Here's how the part is built. I have some questions about the finished solid (model axes, mm). A direction names the side the tool comes from. Round coordinates to 2 decimals unless told otherwise and drop trailing zeros. Write each loop counter-clockwise with the first axis right and the second up, starting at its lowest first coordinate (ties: lowest second). Pieces come first, ordered by that corner, then holes. Notation, with made-up numbers: M -38.5,1 L -13.5,1 A20 ccw -13.5,5 Z; hole C 40,-33 d6. An arc over 180 degrees is marked long. Use one line per item in the form item = value. Start each with the question number.
Q1. We'd pull the mould along Z, two halves only. Please class faces 1 (the face through (40.39, 3.042, -20.515)), 2 (the face through (1, 3, -25)), 3 (the face through (47, 3, -20)), 4 (the face through (-49, 3, 23)): +Z half, -Z half, draft (parallel to the pull), parting line (faces both ways), or undercut.
Q2. I need wall thicknesses on line 1 along X through (y, z) = (4.4, 7); line 2 along X through (y, z) = (2.5, 20); line 3 along Z through (x, y) = (-1, 2.55). Which ranges of each line are inside material? Lowest first, please. Write a range as from..to.
Q3. I want a section at C-C on y = 1.2. List the corners of the cut face in (x, z) for me, and give its area (3 significant figures).
Q4. I want a section at B-B on x = 0. List the corners of the cut face in (y, z) for me, and give its area (3 significant figures).
Q5. I want a section at A-A on z = 0.5. List the corners of the cut face in (x, y) for me, and give its area (3 significant figures).
Q6. For faces 5 (the face through (50, 3, 0)), 6 (the face through (45.515, 3.042, 15.39)), which set-ups out of +Z, -Z, +X, -X, +Y, -Y let a thin tool reach every point of the face, with its end or its side?
Autodesk Inventor part; units mm, degrees
ref_plane "YZ Plane" through (0, 0, 0) normal (1, 0, 0) x (0, 1, 0)
ref_plane "XZ Plane" through (0, 0, 0) normal (0, 1, 0) x (-1, 0, 0)
ref_plane "XY Plane" through (0, 0, 0) normal (0, 0, 1) x (1, 0, 0)
sketch "Sketch1" plane through (0, 0, 0) normal (0, 1, 0) x (-1, 0, 0)
  line L0 (50, 25) -> (-50, 25)
  line L1 (-50, 25) -> (-50, -25)
  line L2 (-50, -25) -> (50, -25)
  line L3 (50, -25) -> (50, 25)
  line L4 (50, 25) -> (-50, -25) construction
  line L5 (-50, 25) -> (50, -25) construction
  point P0 (0, 0)
  dimension "d0" = 100
  dimension "d1" = 50
extrude "Extrusion1" add sketch "Sketch1" along normal blind 6
fillet "Fillet1" radius 5 4 edges at (50, 3, 25) (50, 3, -25) (-50, 3, -25) (-50, 3, 25)
sketch "Sketch2" plane through (0, 6, 0) normal (0, 1, 0) x (1, 0, 0)
  line L0 (-39.5, -21.25) -> (-30.5, -21.25)
  line L1 (-30.5, -21.25) -> (-30.5, -4.75)
  line L2 (-30.5, -4.75) -> (-39.5, -4.75)
  line L3 (-39.5, -4.75) -> (-39.5, -21.25)
  line L4 (-39.5, -21.25) -> (-30.5, -4.75) construction
  line L5 (-30.5, -21.25) -> (-39.5, -4.75) construction
  line L6 (-25.5, -21.25) -> (-16.5, -21.25)
  line L7 (-16.5, -21.25) -> (-16.5, -4.75)
  line L8 (-16.5, -4.75) -> (-25.5, -4.75)
  line L9 (-25.5, -4.75) -> (-25.5, -21.25)
  line L10 (-25.5, -21.25) -> (-16.5, -4.75) construction
  line L11 (-16.5, -21.25) -> (-25.5, -4.75) construction
  line L12 (-11.5, -21.25) -> (-2.5, -21.25)
  line L13 (-2.5, -21.25) -> (-2.5, -4.75)
  line L14 (-2.5, -4.75) -> (-11.5, -4.75)
  line L15 (-11.5, -4.75) -> (-11.5, -21.25)
  line L16 (-11.5, -21.25) -> (-2.5, -4.75) construction
  line L17 (-2.5, -21.25) -> (-11.5, -4.75) construction
  line L18 (2.5, -21.25) -> (11.5, -21.25)
  line L19 (11.5, -21.25) -> (11.5, -4.75)
  line L20 (11.5, -4.75) -> (2.5, -4.75)
  line L21 (2.5, -4.75) -> (2.5, -21.25)
  line L22 (2.5, -21.25) -> (11.5, -4.75) construction
  line L23 (11.5, -21.25) -> (2.5, -4.75) construction
  line L24 (16.5, -21.25) -> (25.5, -21.25)
  line L25 (25.5, -21.25) -> (25.5, -4.75)
  line L26 (25.5, -4.75) -> (16.5, -4.75)
  line L27 (16.5, -4.75) -> (16.5, -21.25)
  line L28 (16.5, -21.25) -> (25.5, -4.75) construction
  line L29 (25.5, -21.25) -> (16.5, -4.75) construction
  line L30 (30.5, -21.25) -> (39.5, -21.25)
  line L31 (39.5, -21.25) -> (39.5, -4.75)
  line L32 (39.5, -4.75) -> (30.5, -4.75)
  line L33 (30.5, -4.75) -> (30.5, -21.25)
  line L34 (30.5, -21.25) -> (39.5, -4.75) construction
  line L35 (39.5, -21.25) -> (30.5, -4.75) construction
  point P0 (0, 0)
  point P1 (-35, -13)
  point P2 (-21, -13)
  point P3 (-7, -13)
  point P4 (7, -13)
  point P5 (21, -13)
  point P6 (35, -13)
  dimension "d5" = 9
  dimension "d6" = 16.5
  dimension "d9" = 14
  dimension "d14" = 7
  dimension "d15" = 13
extrude "Extrusion2" [suppressed]
sketch "Sketch3" plane through (0, 6, 0) normal (0, 1, 0) x (1, 0, 0)
  line L0 (-16.5, -21.25) -> (-25.5, -21.25)
  line L1 (-45, -25) -> (45, -25)
  line L2 (45, 25) -> (-45, 25)
  line L3 (-38, 1) -> (-32, 1)
  line L4 (-32, 1) -> (-32, 21)
  line L5 (-32, 21) -> (-38, 21)
  line L6 (-38, 21) -> (-38, 1)
  line L7 (-38, 1) -> (-32, 21) construction
  line L8 (-32, 1) -> (-38, 21) construction
  line L9 (-24, 1) -> (-18, 1)
  line L10 (-18, 1) -> (-18, 21)
  line L11 (-18, 21) -> (-24, 21)
  line L12 (-24, 21) -> (-24, 1)
  line L13 (-24, 1) -> (-18, 21) construction
  line L14 (-18, 1) -> (-24, 21) construction
  line L15 (-10, 1) -> (-4, 1)
  line L16 (-4, 1) -> (-4, 21)
  line L17 (-4, 21) -> (-10, 21)
  line L18 (-10, 21) -> (-10, 1)
  line L19 (-10, 1) -> (-4, 21) construction
  line L20 (-4, 1) -> (-10, 21) construction
  line L21 (4, 1) -> (10, 1)
  line L22 (10, 1) -> (10, 21)
  line L23 (10, 21) -> (4, 21)
  line L24 (4, 21) -> (4, 1)
  line L25 (4, 1) -> (10, 21) construction
  line L26 (10, 1) -> (4, 21) construction
  line L27 (18, 1) -> (24, 1)
  line L28 (24, 1) -> (24, 21)
  line L29 (24, 21) -> (18, 21)
  line L30 (18, 21) -> (18, 1)
  line L31 (18, 1) -> (24, 21) construction
  line L32 (24, 1) -> (18, 21) construction
  line L33 (32, 1) -> (38, 1)
  line L34 (38, 1) -> (38, 21)
  line L35 (38, 21) -> (32, 21)
  line L36 (32, 21) -> (32, 1)
  line L37 (32, 1) -> (38, 21) construction
  line L38 (38, 1) -> (32, 21) construction
  point P0 (0, 0)
  point P1 (-35, 11)
  point P2 (-21, 11)
  point P3 (-7, 11)
  point P4 (7, 11)
  point P5 (21, 11)
  point P6 (35, 11)
  dimension "d20" = 14
  dimension "d25" = 7
  dimension "d26" = 6
  dimension "d27" = 20
  dimension "d28" = 4
  dimension "d29" = 3.75
extrude "Extrusion3" [suppressed]
sketch "Sketch4" plane through (0, 6, 0) normal (0, 1, 0) x (1, 0, 0)
  arc A0 (-50, -20) -> (-45, -25) centre (-45, -20) ccw
  arc A1 (45, -25) -> (50, -20) centre (45, -20) ccw
  arc A2 (50, 20) -> (45, 25) centre (45, 20) ccw
  arc A3 (-45, 25) -> (-50, 20) centre (-45, 20) ccw
  point P0 (0, 0)
hole "Hole1" at (-45, 6, -20) at (45, 6, -20) at (45, 6, 20) at (-45, 6, 20) direction (0, -1, 0) diameter 4 end through all
sketch "Sketch5" plane through (0, 6, 0) normal (0, 1, 0) x (1, 0, 0)
  circle A0 centre (45, -20) radius 2
  circle A1 centre (-45, 20) radius 2
  circle A2 centre (45, 20) radius 2
  circle A3 centre (-45, -20) radius 2
  line L0 (24, 21) -> (24, 1)
  line L1 (24, 1) -> (18, 1)
  line L2 (18, 1) -> (18, 21)
  line L3 (18, 21) -> (24, 21)
  line L4 (-4, 21) -> (-4, 1)
  line L5 (-4, 1) -> (-10, 1)
  line L6 (-10, 1) -> (-10, 21)
  line L7 (-10, 21) -> (-4, 21)
  line L8 (-32, 21) -> (-32, 1)
  line L9 (-32, 1) -> (-38, 1)
  line L10 (-38, 1) -> (-38, 21)
  line L11 (-38, 21) -> (-32, 21)
  line L12 (-18, 21) -> (-18, 1)
  line L13 (-18, 1) -> (-24, 1)
  line L14 (-24, 1) -> (-24, 21)
  line L15 (-24, 21) -> (-18, 21)
  line L16 (10, 21) -> (10, 1)
  line L17 (10, 1) -> (4, 1)
  line L18 (4, 1) -> (4, 21)
  line L19 (4, 21) -> (10, 21)
  line L20 (38, 21) -> (38, 1)
  line L21 (38, 1) -> (32, 1)
  line L22 (32, 1) -> (32, 21)
  line L23 (32, 21) -> (38, 21)
  line L24 (-45, -25) -> (45, -25)
  line L25 (50, -20) -> (50, 20)
  line L26 (45, 25) -> (-45, 25)
  line L27 (-50, 20) -> (-50, -20)
  line L28 (-39.0839, 21) -> (39.0839, 21)
  line L29 (-46, -14.0839) -> (-46, 14.0839)
  arc A4 (-44.3333, 16.0559) -> (-41.0559, 19.3333) centre (-45, 20) ccw
  arc A5 (41.0559, 19.3333) -> (44.3333, 16.0559) centre (45, 20) ccw
  arc A6 (44.3333, -16.0559) -> (41.0559, -19.3333) centre (45, -20) ccw
  arc A7 (-41.0559, -19.3333) -> (-44.3333, -16.0559) centre (-45, -20) ccw
  line L30 (46, 14.0839) -> (46, -14.0839)
  line L31 (39.0839, -21) -> (-39.0839, -21)
  arc A8 (41.0559, 19.3333) -> (39.0839, 21) centre (39.0839, 19) ccw
  arc A9 (46, 14.0839) -> (44.3333, 16.0559) centre (44, 14.0839) ccw
  arc A10 (44.3333, -16.0559) -> (46, -14.0839) centre (44, -14.0839) ccw
  arc A11 (39.0839, -21) -> (41.0559, -19.3333) centre (39.0839, -19) ccw
  arc A12 (-41.0559, -19.3333) -> (-39.0839, -21) centre (-39.0839, -19) ccw
  arc A13 (-46, -14.0839) -> (-44.3333, -16.0559) centre (-44, -14.0839) ccw
  arc A14 (-39.0839, 21) -> (-41.0559, 19.3333) centre (-39.0839, 19) ccw
  arc A15 (-44.3333, 16.0559) -> (-46, 14.0839) centre (-44, 14.0839) ccw
  point P0 (0, 0)
  point P1 (41.127, 21)
  point P2 (41.127, -21)
  point P3 (-46, -16.127)
  point P4 (-46, 16.127)
  point P5 (46, 16.127)
  point P6 (46, -16.127)
  point P7 (-41.127, -21)
  point P8 (-41.127, 21)
  dimension "d39" = 4
  dimension "d40" = 8
  dimension "d41" = 8
  dimension "d42" = 8
  dimension "d43" = 8
  dimension "d44" = 4
  dimension "d45" = 4
  dimension "d46" = 4
  dimension "d47" = 2
extrude "Extrusion4" cut sketch "Sketch5" against normal blind 10 contours L28 L22 L21 L20 A8 A5 A9 L30 A10 A6 A11 L31 A12 A7 A13 L29 A15 A4 A14 L10 L9 L8 L14 L13 L12 L6 L5 L4 L18 L17 L16 L2 L1 L0 | L0 L1 L2 L3 | L23 L20 L21 L22 | L16 L17 L18 L19 | L4 L5 L6 L7 | L12 L13 L14 L15 | L8 L9 L10 L11
properties part number "AcrylicLowerCore" material "Acrylic, Clear"
Reported:
q1.face_1 = undercut
q1.face_2 = -Z half
q1.face_3 = undercut
q1.face_4 = +Z half
q2.line_1 = -50..-46, 46..50
q2.line_2 = -50..-47, -43..-40.82, 40.82..43, 47..50
q2.line_3 = -25..-21, 21..25
q3.outline = M -50,-20 A5 ccw -45,-25 L 45,-25 A5 ccw 50,-20 L 50,20 A5 ccw 45,25 L -45,25 A5 ccw -50,20 Z; hole C -45,-20 d4; hole C -45,20 d4; hole M -46,-14.08 A2 ccw -44.33,-16.06 A4 cw -41.06,-19.33 A2 ccw -39.08,-21 L 39.08,-21 A2 ccw 41.06,-19.33 A4 cw 44.33,-16.06 A2 ccw 46,-14.08 L 46,14.08 A2 ccw 44.33,16.06 A4 cw 41.06,19.33 A2 ccw 39.08,21 L -39.08,21 A2 ccw -41.06,19.33 A4 cw -44.33,16.06 A2 ccw -46,14.08 Z; hole C 45,-20 d4; hole C 45,20 d4
q3.area = 1,160 mm^2
q4.outline = M 0,-25 L 6,-25 L 6,-21 L 0,-21 Z; M 0,21 L 6,21 L 6,25 L 0,25 Z
q4.area = 48.0 mm^2
q5.outline = M -50,0 L -46,0 L -46,6 L -50,6 Z; M 46,0 L 50,0 L 50,6 L 46,6 Z
q5.area = 48.0 mm^2
q6.face_5 = +Z, -Z, +X, +Y, -Y
q6.face_6 = +Y, -Y
